from build123d import *

# Parameters (mm, degrees)
F0_W     = 30
F0_H     = 30
F1_DEPTH = 30
F2_R     = 5
F3_DEPTH = 30
F4_R     = 2.5
F5_DEPTH = 60.001


with BuildPart() as f1:
    # F0 (on Top) → F1 (new body)
    with BuildSketch(Plane.XY):
        Rectangle(F0_W, F0_H)
    extrude(amount=F1_DEPTH)

    # F2 (on face) → F3 (join)
    with BuildSketch(Plane.XY.offset(30)):
        Circle(F2_R)
    extrude(amount=F3_DEPTH)

    # F4 (on face) → F5 (cut, through all)
    with BuildSketch(Plane.XY.offset(60)):
        Circle(F4_R)
    extrude(amount=-F5_DEPTH, mode=Mode.SUBTRACT)


solid = f1.part
Work out the finished part from the listing and answer in its coordinate system (mm). A direction names the side the tool comes from. Round coordinates to 2 decimals unless told otherwise and drop trailing zeros. Order: outer loops, then holes, each group sorted by start corner. A loop starts at its lowest first (then second) coordinate and runs counter-clockwise, first axis right, second up. Notation, with made-up numbers: M -6,-4.5 L 19,-4.5 A17 ccw 19,22.5 Z; hole C 89.25,43.5 d7. An arc over 180 degrees is marked long. Put each result on its own line as item: value. Start each with the question number.
Q1. Section C-C, the plane z = 5 is taken. Write down the section's boundary in (x, y), and give its area (3 significant figures).
Q2. A tool of negligible diameter and unlimited length cuts with its end or side. For faces 1 (the flat face through (2, -2, 60)), 2 (the flat face through (-4, 4, 30)), from which of +Z, -Z, +X, -X, +Y, -Y can it reach the whole face along a straight path? Write none if from no direction.
Q3. Section A-A, the plane x = 0 is taken. Write down the section's boundary in (y, z).
Q4. Flat-ended cylindrical pins translate along their axes: pin 1 (1.5 mm diameter, centred on x = 0, z = 38, fed in from +Y); pin 2 (2 mm diameter, centred on x = 0, z = 34, fed in from -Y); pin 3 (5 mm diameter, centred on y = -5.5, z = 42.5, fed in from -X). Find the tip coordinate at first contact, or state that the pin passes through.
Q5. For a pull along Y with two mould halves and no side action, classify faces 3 (the flat face through (0, 15, 15)), 4 (the cylindrical face through (-0.54, -2.44, 30.42)), 5 (the flat face through (0, -15, 15)), 6 (the flat face through (-15, 0, 15)) as pulls with the +Y half, pulls with the -Y half, needs draft (parallel to the pull), parting line crosses it, or undercut.
Q6. Straight lines are drawn through the part: L1, parallel to Y at x = 0, z = 13; L2, parallel to Y at x = -0.25, z = 39; L3, parallel to Z at x = 8.75, y = 8.75. For each, find the intervals that lie inside material, in ascending order. Write a range as [from, to].
Q7. Section D-D, the plane x = -6 is taken. Write down the section's boundary in (y, z), and give its area (3 significant figures).
Findings below:
1. outline: M -15,-15 L 15,-15 L 15,15 L -15,15 Z; hole C 0,0 d5
1. area: 880 mm^2
2. face 1: +Z, +X, -X, +Y, -Y
2. face 2: +Z
3. outline: M -15,0 L -2.5,0 L -2.5,60 L -5,60 L -5,30 L -15,30 Z; M 2.5,0 L 15,0 L 15,30 L 5,30 L 5,60 L 2.5,60 Z
4. pin 1: stops at y = 5
4. pin 2: stops at y = -5
4. pin 3: stops at x = -4
5. face 3: pulls with the +Y half
5. face 4: undercut
5. face 5: pulls with the -Y half
5. face 6: needs draft
6. L1: y = [-15, -2.5], [2.5, 15]
6. L2: y = [-4.99, -2.49], [2.49, 4.99]
6. L3: z = [0, 30]
7. outline: M -15,0 L 15,0 L 15,30 L -15,30 Z
7. area: 900 mm^2
